```python
from build123d import *

# Parameters (mm, degrees)
ESBO_O1_R                      = 1.5
RESSALTO_EXTRUS_O1_DEPTH       = 6
ESBO_O6_W                      = 14
ESBO_O6_H                      = 22
RESSALTO_EXTRUS_O3_DEPTH       = 12
ESBO_O7_R                      = 5
CORTE_EXTRUS_O4_DEPTH          = 30.538450843
FILETE3_R                      = 5
ESBO_O11_R                     = 2.5
RESSALTO_EXTRUS_O11_DEPTH      = 6
RESSALTO_EXTRUS_O13_DEPTH      = 8
RESSALTO_EXTRUS_O13_DEPTH_BACK = 5
ESBO_O15_R                     = 2
ESBO_O17_R                     = 1
CORTE_EXTRUS_O6_DEPTH          = 8
ESBO_O20_R                     = 0.75
CORTE_EXTRUS_O7_DEPTH          = 5
ESBO_O21_W                     = 22.669500521
ESBO_O21_H                     = 31.157259519
CORTE_EXTRUS_O8_DEPTH          = 6
ESBO_O22_W                     = 5
ESBO_O22_H                     = 5
ESBO_O22_R                     = 1.5
RESSALTO_EXTRUS_O15_DEPTH      = 3
CHANFRO5_SIZE                  = 1
ESBO_O23_R                     = 1.5
CORTE_EXTRUS_O9_DEPTH          = 17


with BuildPart() as part:
    # Esboço1 → Ressalto-extrusão1 (new body)
    with BuildSketch(Plane.XY):
        Polygon((-10.637137788, -1.832768542), (6.362862212, -1.832768542), (6.362862212, 7.667231458), (10.362862212, 7.667231458), (10.362862212, 16.667231458), (5.362862212, 16.667231458), (5.362862212, 20.167231458), (-10.637137788, 20.167231458), (-10.637137788, 16.667231458), (-15.637137788, 16.667231458), (-15.637137788, 7.667231458), (-10.637137788, 7.667231458), align=None)
        with Locations((6.362862212, 11.867231458)):
            Circle(ESBO_O1_R, mode=Mode.SUBTRACT)
        with Locations((-11.637137788, 11.867231458)):
            Circle(ESBO_O1_R, mode=Mode.SUBTRACT)
    extrude(amount=RESSALTO_EXTRUS_O1_DEPTH)

    # Esboço6 → Ressalto-extrusão3 (add)
    with BuildSketch(Plane(origin=(0, 0, 0), x_dir=(-1, 0, 0), z_dir=(0, 0, -1))):
        with Locations((2.637137788, 9.167231458)):
            Rectangle(ESBO_O6_W, ESBO_O6_H)
    extrude(amount=RESSALTO_EXTRUS_O3_DEPTH)

    # Esboço7 → Corte-extrusão4 (cut, through all)
    with BuildSketch(Plane.XZ.offset(1.832768542)):
        with Locations(Location((-2.637137788, -5, 0), (0, 0, 270))):
            Circle(ESBO_O7_R)
    extrude(amount=-CORTE_EXTRUS_O4_DEPTH, mode=Mode.SUBTRACT)

    # Filete3
    filete3_edges = [part.edges().sort_by_distance(p)[0] for p in [
        (4.362862212, 9.167231458, -12),
        (-9.637137788, 9.167231458, -12),
    ]]
    fillet(filete3_edges, radius=FILETE3_R)

    # Esboço11 → Ressalto-extrusão11 (add)
    with BuildSketch(Plane.XZ.offset(1.832768542)):
        with Locations(Location((3.938862212, 2.7, 0), (0, 0, 14.163833683))):
            Circle(ESBO_O11_R)
    extrude(amount=RESSALTO_EXTRUS_O11_DEPTH)

    # Esboço15 → Ressalto-extrusão13 (add, two sides: drawn at the far end of the back side and taken through both)
    with BuildSketch(Plane(origin=(0, 20.167231458, 0), x_dir=(1, 0, 0), z_dir=(0, 1, 0)).offset(-RESSALTO_EXTRUS_O13_DEPTH_BACK)):
        with Locations(Location((-8.650480796, 5, 0), (0, 0, 270))):
            Circle(ESBO_O15_R)
        with Locations(Location((3.376205221, 5, 0), (0, 0, 270))):
            Circle(ESBO_O15_R)
    extrude(amount=RESSALTO_EXTRUS_O13_DEPTH + RESSALTO_EXTRUS_O13_DEPTH_BACK)

    # Esboço17 → Corte-extrusão6 (cut)
    with BuildSketch(Plane(origin=(0, 28.167231458, 0), x_dir=(1, 0, 0), z_dir=(0, 1, 0))):
        with Locations(Location((-8.650480796, 5, 0), (0, 0, 270))):
            Circle(ESBO_O17_R)
        with Locations(Location((3.376205221, 5, 0), (0, 0, 270))):
            Circle(ESBO_O17_R)
    extrude(amount=-CORTE_EXTRUS_O6_DEPTH, mode=Mode.SUBTRACT)

    # Esboço20 → Corte-extrusão7 (cut)
    with BuildSketch(Plane.XZ.offset(7.832768542)):
        with Locations(Location((3.938862212, 2.7, 0), (0, 0, 270))):
            Circle(ESBO_O20_R)
    extrude(amount=-CORTE_EXTRUS_O7_DEPTH, mode=Mode.SUBTRACT)

    # Esboço21 → Corte-extrusão8 (cut)
    with BuildSketch(Plane(origin=(0, 0, -7.115225733), x_dir=(1, 0, 0), z_dir=(0, 0, -1))):
        with Locations((-2.778124877, -9.864448806)):
            Rectangle(ESBO_O21_W, ESBO_O21_H)
    extrude(amount=CORTE_EXTRUS_O8_DEPTH, mode=Mode.SUBTRACT)

    # Esboço22 → Ressalto-extrusão15 (add)
    # profile 1 of 2: a face of its own
    with BuildSketch(Plane(origin=(0, 0, -7.115225733), x_dir=(1, 0, 0), z_dir=(0, 0, -1))):
        with Locations((-12.135809914, -15.625880271)):
            Rectangle(ESBO_O22_W, ESBO_O22_H)
        with Locations(Location((-12.135809914, -15.625880271, 0), (0, 0, 180))):
            Circle(ESBO_O22_R, mode=Mode.SUBTRACT)
    # profile 2 of 2: a face of its own
    with BuildSketch(Plane(origin=(0, 0, -7.115225733), x_dir=(1, 0, 0), z_dir=(0, 0, -1))):
        with Locations((6.862862212, -15.625880271)):
            Rectangle(ESBO_O22_W, ESBO_O22_H)
        with Locations(Location((6.862862212, -15.625880271, 0), (0, 0, 180))):
            Circle(ESBO_O22_R, mode=Mode.SUBTRACT)
    extrude(amount=-RESSALTO_EXTRUS_O15_DEPTH)

    # Chanfro5
    # the kernel refuses this chamfer: 1 mm, written as the material it takes off along each edge
    with BuildSketch(Plane(origin=(6.362862212, 11.867231458, 0), x_dir=(1, 0, 0), z_dir=(0, -1, 0))) as chanfro5_piece_1_section:
        Polygon((1.5 + CHANFRO5_SIZE, 0), (1.5, CHANFRO5_SIZE), (1.5, 0), align=None)
    chanfro5_piece_1 = revolve(axis=Axis((6.362862212, 11.867231458, 0), (0, 0, 1)), mode=Mode.PRIVATE)
    chanfro5_piece_1 = split(chanfro5_piece_1, bisect_by=Plane(origin=(4.362862212, 13.893105183, 0.134898453), z_dir=(1, 0, 0)), keep=Keep.TOP, mode=Mode.PRIVATE)
    add(chanfro5_piece_1, mode=Mode.SUBTRACT)
    with BuildSketch(Plane(origin=(-11.637137788, 11.867231458, 0), x_dir=(1, 0, 0), z_dir=(0, -1, 0))) as chanfro5_piece_2_section:
        Polygon((1.5 + CHANFRO5_SIZE, 0), (1.5, CHANFRO5_SIZE), (1.5, 0), align=None)
    chanfro5_piece_2 = revolve(axis=Axis((-11.637137788, 11.867231458, 0), (0, 0, 1)), mode=Mode.PRIVATE)
    chanfro5_piece_2 = split(chanfro5_piece_2, bisect_by=Plane(origin=(-9.637137788, 11.867231458, 0.487087965), z_dir=(-1, 0, 0)), keep=Keep.TOP, mode=Mode.PRIVATE)
    add(chanfro5_piece_2, mode=Mode.SUBTRACT)

    # Esboço23 → Corte-extrusão9 (cut)
    with BuildSketch(Plane.ZY.offset(9.637137788)):
        with Locations((-1.5, 16.167231458)):
            Circle(ESBO_O23_R)
    extrude(amount=-CORTE_EXTRUS_O9_DEPTH, mode=Mode.SUBTRACT)


solid = part.part
```
Build history of the part. All positions in model axes, mm. A direction names the side the tool comes from. Coordinates: 2 decimals unless noted, no trailing zeros. Write each loop counter-clockwise with the first axis right and the second up, starting at its lowest first coordinate (ties: lowest second). Pieces come first, ordered by that corner, then holes.
1. Pull direction X, two halves, no side cores. Call faces 1 (the cylindrical face through (6.07, -4.79, 4.01)), 2 (the flat face through (8, 16.667, 3)), 3 (the cylindrical face through (-12.827, 10.955, 3.465)): released by +X, released by -X, zero draft, split by the parting line, or undercut.
Answer block:
face 1: split by the parting line
face 2: zero draft
face 3: undercut
2. Band-saw the part on B-B, the plane z = 2.7. Give the cut face in (x, y).
Answer block:
outline: (-15.64, 7.67) - (-10.64, 7.67) - (-10.64, -1.83) - (1.44, -1.83) - (1.44, -7.83) - (3.19, -7.83) - (3.19, -2.83) - (4.69, -2.83) - (4.69, -7.83) - (6.44, -7.83) - (6.44, -1.83) - (6.36, -1.83) - (6.36, 7.67) - (10.36, 7.67) - (10.36, 16.67) - (5.36, 16.67) - (5.36, 20.17) - (-10.64, 20.17) - (-10.64, 16.67) - (-15.64, 16.67) - close; hole circle Ø3 at (-11.64, 11.87); hole circle Ø3 at (6.36, 11.87)
3. Band-saw the part on A-A, the plane y = -1. Give the cut face in (x, z).
Answer block:
outline: (-10.64, 0) - (-9.64, 0) - (-9.64, -7) arc R5 ccw to (-9.64, -7.12) - (-7.17, -7.12) arc R5 cw (long way) to (1.89, -7.12) - (4.36, -7.12) arc R5 ccw to (4.36, -7) - (4.36, 0) - (6.36, 0) - (6.36, 6) - (-10.64, 6) - close
4. Drop flat-ended pins along their axis: pin 1 (4 mm diameter, centred on y = 14, z = -4, fed in from +X); pin 2 (1.2 mm diameter, centred on x = 3.38, z = -5, fed in from +Y); pin 3 (1 mm diameter, centred on y = 6, z = 4, fed in from -X). Give the stop position or say it passes through.
Answer block:
pin 1: stops at x = 9.36
pin 2: stops at y = 20.17
pin 3: stops at x = -10.64
5. Band-saw the part on C-C, the plane z = -1.5. Give the cut face in (x, y).
Answer block:
outline: (-9.64, -1.83) - (-6.21, -1.83) - (-6.21, 14.67) - (-9.64, 14.67) - close; (-9.64, 17.67) - (-6.21, 17.67) - (-6.21, 20.17) - (-9.64, 20.17) - close; (0.93, -1.83) - (4.36, -1.83) - (4.36, 14.67) - (0.93, 14.67) - close; (0.93, 17.67) - (4.36, 17.67) - (4.36, 20.17) - (0.93, 20.17) - close
6. 3-axis set-ups, long thin cutter, end or side, ignore diameter. For faces 4 (the flat face through (4.7, 15.167, -3.8)), 5 (the conical face through (7.896, 11.232, 0.84)), 6 (the cylindrical face through (-6.668, 23.021, -5.26)), 7 (the flat face through (7, 13.126, -6)): which of +Z, -Z, +X, -X, +Y, -Y reach the whole face in a straight line?
Answer block:
face 4: +X, -Y
face 5: none
face 6: +Y
face 7: -Z, +X, -Y
7. Drill centre lines: probe 1 along X at (y, z) = (12, 3.5); probe 2 along X at (y, z) = (-4, 2.7); probe 3 along X at (y, z) = (6.5, -5). Where is each one in solid material? Low to high.
Answer block:
probe 1: x = -15.64 to -13.13, -10.14 to 4.87, 7.86 to 10.36
probe 2: x = 1.44 to 3.19, 4.69 to 6.44
probe 3: x = -9.64 to -7.64, 2.36 to 4.36
